Source: CAD feature listing. Evaluate the final solid. Frame: model axes, mm. Face numbers are marked on the shaded views. A direction names the side the tool comes from. Round coordinates to 2 decimals unless told otherwise and drop trailing zeros. Order: outer loops, then holes, each group sorted by start corner. A loop starts at its lowest first (then second) coordinate and runs counter-clockwise, first axis right, second up. Notation, with made-up numbers: M 43.5,-9.75 L 69.5,-9.75 A36 cw 69.5,29.25 Z; hole C 65.5,2 d4. An arc over 180 degrees is marked long. Answer in a Markdown table with one row per item. Add a question column.
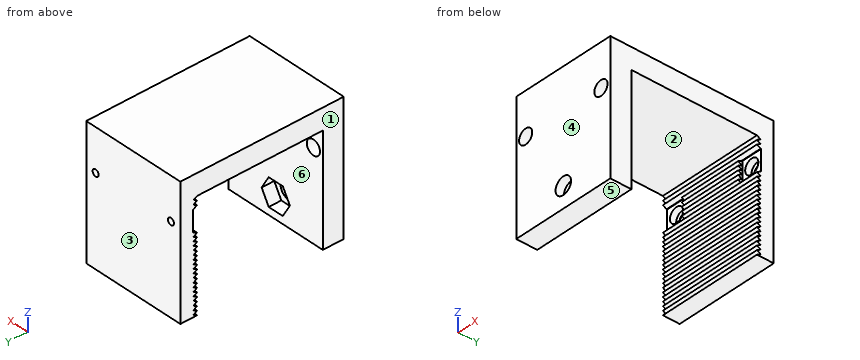
```python
from build123d import *

# Parameters (mm, degrees)
SKETCH1_W               = 50
SKETCH1_H               = 62
BOSS_EXTRUDE1_DEPTH     = 8
SKETCH2_R               = 1.6
CUT_EXTRUDE1_DEPTH      = 41.620192023
SKETCH4_W               = 50
SKETCH4_H               = 10
BOSS_EXTRUDE2_DEPTH     = 60
SKETCH5_W               = 50
SKETCH5_H               = 62
BOSS_EXTRUDE3_DEPTH     = 10
SKETCH6_R               = 4.1
CUT_EXTRUDE3_DEPTH      = 10
CUT_EXTRUDE4_START      = -50
CUT_EXTRUDE4_DEPTH      = 50
CUT_EXTRUDE6_DEPTH      = 6
CUT_EXTRUDE7_START      = -8
SKETCH10_W              = 10
SKETCH10_H              = 10
CUT_EXTRUDE7_DEPTH      = 2
CUT_EXTRUDE8_DEPTH      = 83.280009723
CUT_EXTRUDE8_DEPTH_BACK = 3
SKETCH11_R              = 3.5


# Read off the part's stored shape, not the designer's step: Cut-Extrude4
with BuildPart() as part:
    # Sketch1 → Boss-Extrude1 (new body)
    with BuildSketch(Plane(origin=(0, 0, 0), x_dir=(1, 0, 0), z_dir=(0, 1, 0))):
        Rectangle(SKETCH1_W, SKETCH1_H)
    extrude(amount=BOSS_EXTRUDE1_DEPTH)

    # Sketch2 → Cut-Extrude1 (cut, through all)
    with BuildSketch(Plane(origin=(0, 8, 0), x_dir=(1, 0, 0), z_dir=(0, 1, 0))):
        with Locations(Location((-20, -11, 0), (0, 0, 270))):
            Circle(SKETCH2_R)
        with Locations(Location((20, -11, 0), (0, 0, 270))):
            Circle(SKETCH2_R)
    extrude(amount=-CUT_EXTRUDE1_DEPTH, mode=Mode.SUBTRACT)

    # Sketch4 → Boss-Extrude2 (add)
    with BuildSketch(Plane.XZ):
        with Locations((0, 26)):
            Rectangle(SKETCH4_W, SKETCH4_H)
    extrude(amount=BOSS_EXTRUDE2_DEPTH)

    # Sketch5 → Boss-Extrude3 (add)
    with BuildSketch(Plane.XZ.offset(60)):
        Rectangle(SKETCH5_W, SKETCH5_H)
    extrude(amount=BOSS_EXTRUDE3_DEPTH)

    # Sketch6 → Cut-Extrude3 (cut)
    with BuildSketch(Plane.XZ.offset(70)):
        with Locations(Location((0, -21, 0), (0, 0, 270))):
            Circle(SKETCH6_R)
    extrude(amount=-CUT_EXTRUDE3_DEPTH, mode=Mode.SUBTRACT)

    # Cut-Extrude4 outline → Cut-Extrude4 (cut)
    with BuildSketch(Plane.ZY.offset(25).offset(CUT_EXTRUDE4_START)):
        Polygon((20, 1.732050808), (19, 0), (21, 0), align=None)
        Polygon((18, 1.732050808), (17, 0), (19, 0), align=None)
        Polygon((16, 1.732050808), (15, 0), (17, 0), align=None)
        Polygon((14, 1.732050808), (13, 0), (15, 0), align=None)
        Polygon((-31, 0), (-29, 0), (-30, 1.732050808), align=None)
        Polygon((-29, 0), (-27, 0), (-28, 1.732050808), align=None)
        Polygon((-27, 0), (-25, 0), (-26, 1.732050808), align=None)
        Polygon((-25, 0), (-23, 0), (-24, 1.732050808), align=None)
        Polygon((-23, 0), (-21, 0), (-22, 1.732050808), align=None)
        Polygon((-21, 0), (-19, 0), (-20, 1.732050808), align=None)
        Polygon((-19, 0), (-17, 0), (-18, 1.732050808), align=None)
        Polygon((-17, 0), (-15, 0), (-16, 1.732050808), align=None)
        Polygon((-15, 0), (-13, 0), (-14, 1.732050808), align=None)
        Polygon((-13, 0), (-11, 0), (-12, 1.732050808), align=None)
        Polygon((-11, 0), (-9, 0), (-10, 1.732050808), align=None)
        Polygon((-9, 0), (-7, 0), (-8, 1.732050808), align=None)
        Polygon((-7, 0), (-5, 0), (-6, 1.732050808), align=None)
        Polygon((-5, 0), (-3, 0), (-4, 1.732050808), align=None)
        Polygon((-3, 0), (-1, 0), (-2, 1.732050808), align=None)
        Polygon((-1, 0), (1, 0), (0, 1.732050808), align=None)
        Polygon((1, 0), (3, 0), (2, 1.732050808), align=None)
        Polygon((3, 0), (5, 0), (4, 1.732050808), align=None)
        Polygon((5, 0), (7, 0), (6, 1.732050808), align=None)
        Polygon((7, 0), (9, 0), (8, 1.732050808), align=None)
        Polygon((9, 0), (11, 0), (10, 1.732050808), align=None)
        Polygon((13, 0), (12, 1.732050808), (11, 0), align=None)
    extrude(amount=CUT_EXTRUDE4_DEPTH, mode=Mode.SUBTRACT)

    # Sketch9 → Cut-Extrude6 (cut)
    with BuildSketch(Plane(origin=(0, -60, 0), x_dir=(1, 0, 0), z_dir=(0, 1, 0))):
        Polygon((3.75, 14.504809472), (7.5, 21), (3.75, 27.495190528), (-3.75, 27.495190528), (-7.5, 21), (-3.75, 14.504809472), align=None)
    extrude(amount=-CUT_EXTRUDE6_DEPTH, mode=Mode.SUBTRACT)

    # Sketch10 → Cut-Extrude7 (cut)
    with BuildSketch(Plane(origin=(0, 8, 0), x_dir=(1, 0, 0), z_dir=(0, 1, 0)).offset(CUT_EXTRUDE7_START)):
        with Locations((20, -11)):
            Rectangle(SKETCH10_W, SKETCH10_H)
        with Locations((-20, -11)):
            Rectangle(SKETCH10_W, SKETCH10_H)
    extrude(amount=CUT_EXTRUDE7_DEPTH, mode=Mode.SUBTRACT)

    # Sketch11 → Cut-Extrude8 (cut, two sides: drawn at the far end of the back side and taken through both)
    with BuildSketch(Plane.XZ.offset(-2).offset(-CUT_EXTRUDE8_DEPTH_BACK)):
        with Locations(Location((-20, 11, 0), (0, 0, 90))):
            Circle(SKETCH11_R)
        with Locations(Location((20, 11, 0), (0, 0, 90))):
            Circle(SKETCH11_R)
    extrude(amount=CUT_EXTRUDE8_DEPTH + CUT_EXTRUDE8_DEPTH_BACK, mode=Mode.SUBTRACT)


solid = part.part
```
(1) Draft query along Y for the marked faces 3, 4, 5 and 6. Return one class per face: +Y half, -Y half, draft (parallel to the pull), parting line (faces both ways), or undercut.
(2) Pin query (flat end, axial travel): pin 1 (0.6 mm diameter, centred on y = 1.5, z = 10.5, fed in from -X); pin 2 (8 mm diameter, centred on y = -4.5, z = 12, fed in from +X); pin 3 (1 mm diameter, centred on x = 10.5, y = -30, fed in from -Z). Return the tip coordinate at first contact, or that it passes through.
(3) Cut plane A-A (x = -20). Count the separate pieces of the cut face and the enclosed holes in it, and give its area (3 significant figures).
(4) Cut plane B-B (y = -6). Return loops of the section in (x, z), and give its area (3 significant figures).
(5) Line query: line 1 (Z direction, x = 20, y = 4); line 2 (X direction, y = -68.45, z = -21); line 3 (X direction, y = 3, z = 11). Output: solid intervals per line, ascending. Write a range as from..to.
(6) Access query for the marked faces 1 and 2. Directions: +Z, -Z, +X, -X, +Y, -Y. A direction counts if a zero-diameter tool reaches every point of the face in a straight line with its end or side. Return the directions, or none.
Answer list:
| question | item | result |
|---|---|---|
| 1 | face 3 | +Y half |
| 1 | face 4 | -Y half |
| 1 | face 5 | draft |
| 1 | face 6 | undercut |
| 2 | pin 1 | x = -15 |
| 2 | pin 2 | through |
| 2 | pin 3 | z = 21 |
| 3 | separate pieces | 3 |
| 3 | enclosed holes | 0 |
| 3 | area | 1,560 mm² |
| 4 | outline | M -25,21 L 25,21 L 25,31 L -25,31 Z |
| 4 | area | 500 mm² |
| 5 | line 1 | -31..7.5, 14.5..31 |
| 5 | line 2 | -25..-4.1, 4.1..25 |
| 5 | line 3 | -25..-23.5, -16.5..16.5, 23.5..25 |
| 6 | face 1 | +Z, -Z, -X, +Y, -Y |
| 6 | face 2 | -Z, +X, -X |
